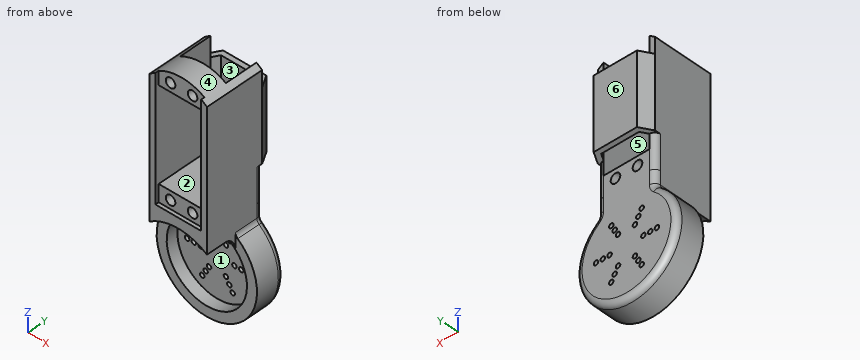
```python
from build123d import *

# Parameters (mm, degrees)
SKETCH2_R           = 22.224999999999998
BOSS_EXTRUDE1_DEPTH = 12.7
SKETCH3_R           = 1.0000000000000009
SKETCH3_R_2         = 1.0000000000000002
SKETCH3_R_3         = 0.9999999999999998
CUT_EXTRUDE1_DEPTH  = 34.89972345019941
BOSS_EXTRUDE2_START = -19.05
BOSS_EXTRUDE2_DEPTH = 19.05
SKETCH8_R           = 17.779999999999998
CUT_EXTRUDE2_DEPTH  = 5.08
FILLET5_R           = 5.08
FILLET6_R           = 2.5399999999999996
FILLET7_R           = 2.5399999999999996
BOSS_EXTRUDE3_START = 7.211059999999999
BOSS_EXTRUDE3_DEPTH = 7.211059999999999
BOSS_EXTRUDE4_DEPTH = 25.4
SKETCH13_W          = 25.399999999999995
SKETCH13_H          = 26.261059999999993
BOSS_EXTRUDE5_DEPTH = 12.7
SKETCH15_W          = 20.32
SKETCH15_H          = 3.8100000000000023
CUT_EXTRUDE3_DEPTH  = 58.77305999999999
SKETCH16_W          = 20.32
SKETCH16_H          = 7.619999999999997
CUT_EXTRUDE4_DEPTH  = 1.5493999999999999
SKETCH18_R          = 2.1259799999999998
SKETCH18_R_2        = 2.12598
CUT_EXTRUDE5_DEPTH  = 38.09999999999998
SKETCH19_W          = 2.5399999999999974
SKETCH19_H          = 26.261059999999993
BOSS_EXTRUDE6_DEPTH = 39.370000000000005
BOSS_EXTRUDE7_DEPTH = 31.75
FILLET12_R          = 2.54
FILLET13_R          = 2.54
BOSS_EXTRUDE8_DEPTH = 10.15999999999999
SKETCH25_R          = 2.1259800000000015
SKETCH25_R_2        = 2.125980000000002
CUT_EXTRUDE6_DEPTH  = 10.15999999999999
BOSS_EXTRUDE9_DEPTH = 26.26106


# Some blends are built 0.0001 mm under size
with BuildPart() as part:
    # Sketch2 → Boss-Extrude1 (new body)
    with BuildSketch(Plane(origin=(0, 0, 0), x_dir=(1, 0, 0), z_dir=(0, 1, 0))):
        with Locations(Location((0, 0, 0), (0, 0, 270))):
            Circle(SKETCH2_R)
    extrude(amount=BOSS_EXTRUDE1_DEPTH)

    # Sketch3 → Cut-Extrude1 (cut, through all)
    with BuildSketch(Plane(origin=(0, 12.7, 0), x_dir=(1, 0, 0), z_dir=(0, 1, 0))):
        with Locations(Location((-6.750000000000055, -11.691342951089895, 0), (0, 0, 270))):
            Circle(SKETCH3_R)
        with Locations(Location((-5.2500000000000435, -9.093266739736585, 0), (0, 0, 270))):
            Circle(SKETCH3_R)
        with Locations(Location((-3.7500000000000306, -6.495190528383274, 0), (0, 0, 270))):
            Circle(SKETCH3_R_2)
        with Locations(Location((-13.5, -9.2e-16, 0), (0, 0, 270))):
            Circle(SKETCH3_R_3)
        with Locations(Location((-10.5, -9.2e-16, 0), (0, 0, 270))):
            Circle(SKETCH3_R_3)
        with Locations(Location((-7.5, -9.2e-16, 0), (0, 0, 270))):
            Circle(SKETCH3_R_3)
        with Locations(Location((-3.7499999999999396, 6.495190528383324, 0), (0, 0, 270))):
            Circle(SKETCH3_R_3)
        with Locations(Location((-5.2499999999999165, 9.093266739736652, 0), (0, 0, 270))):
            Circle(SKETCH3_R)
        with Locations(Location((-6.749999999999892, 11.69134295108998, 0), (0, 0, 270))):
            Circle(SKETCH3_R)
        with Locations(Location((6.750000000000136, 11.69134295108984, 0), (0, 0, 270))):
            Circle(SKETCH3_R)
        with Locations(Location((5.250000000000107, 9.093266739736544, 0), (0, 0, 270))):
            Circle(SKETCH3_R)
        with Locations(Location((3.750000000000076, 6.495190528383245, 0), (0, 0, 270))):
            Circle(SKETCH3_R_2)
        with Locations(Location((13.5, -9.2e-16, 0), (0, 0, 270))):
            Circle(SKETCH3_R_3)
        with Locations(Location((10.5, -9.2e-16, 0), (0, 0, 270))):
            Circle(SKETCH3_R_3)
        with Locations(Location((7.5, -9.2e-16, 0), (0, 0, 270))):
            Circle(SKETCH3_R_3)
        with Locations(Location((3.749999999999985, -6.4951905283833, 0), (0, 0, 270))):
            Circle(SKETCH3_R_2)
        with Locations(Location((5.24999999999998, -9.09326673973662, 0), (0, 0, 270))):
            Circle(SKETCH3_R)
        with Locations(Location((6.749999999999973, -11.69134295108994, 0), (0, 0, 270))):
            Circle(SKETCH3_R)
    extrude(amount=-CUT_EXTRUDE1_DEPTH, mode=Mode.SUBTRACT)

    # Sketch4 → Boss-Extrude2 (add)
    with BuildSketch(Plane(origin=(0, 12.7, 0), x_dir=(1, 0, 0), z_dir=(0, 1, 0)).offset(BOSS_EXTRUDE2_START)):
        with BuildLine():
            Line((-12.7, -18.23898640275824), (-12.7, -25.4))
            Line((-12.7, -25.4), (12.7, -25.4))
            Line((12.7, -25.4), (12.7, -18.23898640275824))
            ThreePointArc((12.7, -18.23898640275824), (1.36e-15, -22.224999999999998), (-12.7, -18.23898640275824))
        make_face()
    extrude(amount=BOSS_EXTRUDE2_DEPTH)

    # Sketch8 → Cut-Extrude2 (cut)
    with BuildSketch(Plane.XZ):
        with Locations(Location((0, 0, 0), (0, 0, 270))):
            Circle(SKETCH8_R)
    extrude(amount=-CUT_EXTRUDE2_DEPTH, mode=Mode.SUBTRACT)

    # Fillet5
    # the kernel refuses this fillet: 5.08 mm, written as the material it adds along each edge
    with BuildSketch(Plane(origin=(0, 0, 0), x_dir=(0.9228165811173926, 0, 0.3852396106513539), z_dir=(0.3852396106513539, 0, -0.9228165811173926))) as fillet5_piece_1_section:
        with BuildLine():
            CenterArc((17.144999999999996, 5.040156247578053), FILLET5_R, 277.1807557814583, 82.81924421854174)
            Line((22.224999999999998, 5.040156247578053), (22.225000000000648, 0))
            Line((22.225000000000648, 0), (17.779999999999994, 7.11e-15))
        make_face()
    fillet5_piece_1 = revolve(axis=Axis((0, 0, 0), (0, -1, 0)), revolution_arc=134.68276722332823, mode=Mode.PRIVATE)
    fillet5_piece_1 = split(fillet5_piece_1, bisect_by=Plane(origin=(-12.7, -1.6733318741959158, 20.962619999999998), z_dir=(1, 0, 0)), keep=Keep.TOP, mode=Mode.PRIVATE)
    fillet5_piece_1 = split(fillet5_piece_1, bisect_by=Plane(origin=(12.7, -1.6733318741959158, 20.962619999999998), z_dir=(-1, 0, 0)), keep=Keep.TOP, mode=Mode.PRIVATE)
    add(fillet5_piece_1)

    # Fillet6
    fillet6_edges = [part.edges().sort_by_distance(p)[0] for p in [
        (-12.699999999999998, 6.35, 18.238986402758243),
        (12.7, 6.35, 18.23898640275824),
    ]]
    fillet(fillet6_edges, radius=FILLET6_R)

    # Fillet7
    fillet7_edges = [part.edges().sort_by_distance(p)[0] for p in [
        (6.8e-15, 12.7, -22.224999999999998),
        (-12.7, 12.7, 22.460220604576516),
        (12.957258732946789, 12.7, 18.406577524633107),
        (-12.957258732946793, 12.7, 18.4065775246331),
        (12.7, 12.7, 22.460220604576516),
    ]]
    fillet(fillet7_edges, radius=FILLET7_R)

    # Sketch9 → Boss-Extrude3 (add)
    with BuildSketch(Plane.XZ.offset(6.350000000000001).offset(BOSS_EXTRUDE3_START)):
        with BuildLine():
            Line((12.699999999999998, 18.238986402758243), (12.7, 25.4))
            Line((12.7, 25.4), (-12.7, 25.4))
            Line((-12.7, 25.4), (-12.699999999999998, 18.23898640275824))
            ThreePointArc((-12.699999999999998, 18.23898640275824), (1.36e-15, 22.225), (12.699999999999998, 18.238986402758243))
        make_face()
    extrude(amount=-BOSS_EXTRUDE3_DEPTH)

    # Sketch10 → Boss-Extrude4 (add)
    with BuildSketch(Plane(origin=(12.7, 0, 0), x_dir=(0, 0, -1), z_dir=(1, 0, 0))):
        Polygon((-25.4, 12.7), (-38.1, -0.8610600000000003), (-38.1, -13.56106), (-25.4, -13.56106), align=None)
    extrude(amount=-BOSS_EXTRUDE4_DEPTH)

    # Sketch13 → Boss-Extrude5 (add)
    with BuildSketch(Plane.XY.offset(38.1)):
        with Locations((0, -0.4305300000000001)):
            Rectangle(SKETCH13_W, SKETCH13_H)
    extrude(amount=-BOSS_EXTRUDE5_DEPTH)

    # Sketch15 → Cut-Extrude3 (cut)
    with BuildSketch(Plane(origin=(0, 12.7, 0), x_dir=(1, 0, 0), z_dir=(0, 1, 0))):
        with Locations((0, -36.195)):
            Rectangle(SKETCH15_W, SKETCH15_H)
    extrude(amount=-CUT_EXTRUDE3_DEPTH, mode=Mode.SUBTRACT)

    # Sketch16 → Cut-Extrude4 (cut)
    with BuildSketch(Plane.XZ.offset(13.56106)):
        with Locations((0, 30.48)):
            Rectangle(SKETCH16_W, SKETCH16_H)
    extrude(amount=-CUT_EXTRUDE4_DEPTH, mode=Mode.SUBTRACT)

    # Sketch18 → Cut-Extrude5 (cut)
    with BuildSketch(Plane.XZ.offset(12.011660000000001)):
        with Locations(Location((-4.8742600000000005, 30.375860000000003, 0), (0, 0, 270))):
            Circle(SKETCH18_R)
        with Locations(Location((4.8742600000000005, 30.375860000000003, 0), (0, 0, 270))):
            Circle(SKETCH18_R_2)
    extrude(amount=-CUT_EXTRUDE5_DEPTH, mode=Mode.SUBTRACT)

    # Sketch19 → Boss-Extrude6 (add)
    with BuildSketch(Plane.XY.offset(38.1)):
        with Locations((-11.43, -0.4305300000000001)):
            Rectangle(SKETCH19_W, SKETCH19_H)
        Polygon((10.16, 12.7), (10.159999999999998, -13.56106), (12.7, -13.56106), (12.7, 12.7), align=None)
    extrude(amount=BOSS_EXTRUDE6_DEPTH)

    # Sketch20 → Boss-Extrude7 (add)
    with BuildSketch(Plane.XY.offset(40.64)):
        Polygon((-12.7, 12.7), (-9.5885, 18.033999999999995), (9.588500000000002, 18.033999999999995), (12.7, 12.7), (10.16, 12.7), (8.382000000000001, 15.747999999999998), (-8.382000000000001, 15.747999999999994), (-10.16, 12.7), align=None)
    extrude(amount=BOSS_EXTRUDE7_DEPTH)

    # Fillet12
    fillet12_edges = [part.edges().sort_by_distance(p)[0] for p in [
        (12.699999999999998, 12.699999999999998, 33.02),
    ]]
    fillet(fillet12_edges, radius=FILLET12_R - 0.0001)  # a hair under: the kernel refuses the full size

    # Fillet13
    fillet13_edges = [part.edges().sort_by_distance(p)[0] for p in [
        (-12.699999999999998, 12.699999999999998, 33.02),
    ]]
    fillet(fillet13_edges, radius=FILLET13_R - 0.0001)  # a hair under: the kernel refuses the full size

    # Sketch24 → Boss-Extrude8 (add)
    with BuildSketch(Plane.XZ.offset(12.011660000000001)):
        with BuildLine():
            Line((-10.16, 75.184), (-10.16, 81.15627063227116))
            ThreePointArc((-10.16, 81.15627063227116), (1.25e-15, 83.87080000000003), (10.159999999999998, 81.15627063227116))
            Line((10.159999999999998, 81.15627063227116), (10.16, 75.184))
            Line((10.16, 75.184), (-10.16, 75.184))
        make_face()
    extrude(amount=-BOSS_EXTRUDE8_DEPTH)

    # Sketch25 → Cut-Extrude6 (cut)
    with BuildSketch(Plane.XZ.offset(12.011660000000001)):
        with Locations(Location((-4.8742600000000005, 78.97622, 0), (0, 0, 270))):
            Circle(SKETCH25_R)
        with Locations(Location((4.874260000000001, 78.97622, 0), (0, 0, 270))):
            Circle(SKETCH25_R_2)
    extrude(amount=-CUT_EXTRUDE6_DEPTH, mode=Mode.SUBTRACT)

    # Sketch26 → Boss-Extrude9 (add)
    with BuildSketch(Plane.XZ.offset(13.56106)):
        with BuildLine():
            ThreePointArc((-12.7, 79.4273190663087), (-11.462644475833708, 80.33975279689817), (-10.16, 81.15627063227114))
            Line((-10.16, 81.15627063227114), (-10.16, 77.47000000000001))
            Line((-10.16, 77.47000000000001), (-12.7, 77.47000000000001))
            Line((-12.7, 77.47000000000001), (-12.7, 79.4273190663087))
        make_face()
        with BuildLine():
            ThreePointArc((12.7, 79.4273190663087), (11.4626444758337, 80.33975279689815), (10.159999999999991, 81.15627063227114))
            Line((10.159999999999998, 81.15627063227116), (10.159999999999998, 77.47000000000001))
            Line((10.159999999999998, 77.47000000000001), (12.7, 77.47000000000001))
            Line((12.7, 77.47000000000001), (12.7, 79.4273190663087))
        make_face()
    extrude(amount=-BOSS_EXTRUDE9_DEPTH)


solid = part.part
```
For this review, take the finished solid that the model builds, in its own axes (mm). Face numbers are marked on the shaded views. A direction names the side the tool comes from. Give positions to 0.01 mm unless a question says otherwise; leave off trailing zeros. Write each loop counter-clockwise with the first axis right and the second up, starting at its lowest first coordinate (ties: lowest second). Pieces come first, ordered by that corner, then holes.
Item 1: Take a section at D-D (y = -3). Give the boundary of the cut face in (x, z), and give its area (3 significant figures).
Item 2: Wall thickness on probe 1 along Z at (x, y) = (5.5, -9); probe 2 along X at (y, z) = (0, 48); probe 3 along Y at (x, z) = (5, 56.5): over which ranges is each line inside the solid? List them lowest first.
Item 3: Take a section at C-C (z = 62). Give the boundary of the cut face in (x, y), and give its area (3 significant figures).
Item 4: Take a section at B-B (x = 0). Give the boundary of the cut face in (y, z) (3 decimals).
Item 5: Machinability: for the marked faces 1, 2 and 3, which of the approach directions +Z, -Z, +X, -X, +Y, -Y give a long, thin tool a straight path to every point of the face, cutting with its end or side? Answer none if there is none.
Item 6: Insertion check: P1, Ø8, axis at x = 2.5, z = 53.5, coming from the -Y side; P2, Ø16.5, axis at x = -0.5, y = 5.5, coming from the +Z side; P3, Ø2.5, axis at x = 4.5, z = 80.5, coming from the -Y side; P4, Ø6, axis at y = 5, z = -2.5, coming from the +X side (3 decimals). Each pin has a flat end and moves straight along its axis. Give the tip position at first contact, or say it passes through.
Item 7: The part is to be moulded in two halves that separate along Z. For the marked faces 4, 5 and 6, say which applies: +Z half, -Z half, draft (parallel to the pull), parting line (faces both ways), or undercut.
Established:
1. outline: (-12.7, 17.72) arc R21.8 cw to (12.7, 17.72) - (12.7, 79.43) arc R20.37 ccw to (-12.7, 79.43) - close; hole (-10.16, 34.29) - (10.16, 34.29) - (10.16, 75.18) - (-10.16, 75.18) - close; hole circle Ø4.25 at (-4.87, 30.38); hole circle Ø4.25 at (-4.87, 78.98); hole circle Ø4.25 at (4.87, 30.38); hole circle Ø4.25 at (4.87, 78.98)
1. area: 686 mm2
2. probe 1: z = 21.53 to 28.34, 32.41 to 34.29, 75.18 to 76.94, 81.01 to 83.11
2. probe 2: x = -12.7 to -10.16, 10.16 to 12.7
2. probe 3: y = 15.75 to 18.03
3. outline: (-12.7, -13.56) - (-10.16, -13.56) - (-10.16, 12.7) - (-8.38, 15.75) - (8.38, 15.75) - (10.16, 12.7) - (10.16, -13.56) - (12.7, -13.56) - (12.7, 12.7) - (9.59, 18.03) - (-9.59, 18.03) - (-12.7, 12.7) - close
3. area: 196 mm2
4. outline: (-13.561, 22.225) - (-5.04, 22.225) arc R5.08 cw to (0, 17.78) - (5.08, 17.78) - (5.08, -17.78) - (0, -17.78) - (0, -22.225) - (10.16, -22.225) arc R2.54 ccw to (12.7, -19.685) - (12.7, 34.29) - (-12.012, 34.29) - (-12.012, 26.67) - (-13.561, 26.67) - close; (-12.012, 75.184) - (-1.852, 75.184) - (-1.852, 83.871) - (-12.012, 83.871) - close; (15.748, 40.64) - (18.034, 40.64) - (18.034, 72.39) - (15.748, 72.39) - close
5. face 1: -Y
5. face 2: +Y, -Y
5. face 3: +Z, -Z, -Y
6. P1: stops at y = 15.75
6. P2: stops at z = 83.87
6. P3: stops at y = -12.01
6. P4: stops at x = 22.225
7. face 4: +Z half
7. face 5: undercut
7. face 6: draft
